```python
from build123d import *

# Parameters (mm, degrees)
F0_W     = 99
F0_H     = 38
F0_W_2   = 29.5
F0_H_2   = 16
F1_DEPTH = 3
F2_R     = 2.38125
F3_DEPTH = 3.001
F4_W     = 35.15
F4_H     = 22.55
F5_DEPTH = 1


with BuildPart() as f1:
    # F0 (on Top) → F1 (new body)
    with BuildSketch(Plane.XY):
        with Locations((49.5, 19)):
            Rectangle(F0_W, F0_H)
        with Locations((49.5, 19)):
            Rectangle(F0_W_2, F0_H_2, mode=Mode.SUBTRACT)
    extrude(amount=F1_DEPTH)

    # F2 (on face) → F3 (cut, through all)
    with BuildSketch(Plane.XY.offset(3)):
        with Locations((7.5, 19)):
            Circle(F2_R)
        with Locations((91.5, 19)):
            Circle(F2_R)
    extrude(amount=-F3_DEPTH, mode=Mode.SUBTRACT)

    # F4 (on face) → F5 (cut)
    with BuildSketch(Plane(origin=(0, 0, 0), x_dir=(1, 0, 0), z_dir=(0, 0, -1))):
        with Locations((49.5, -19)):
            Rectangle(F4_W, F4_H)
    extrude(amount=-F5_DEPTH, mode=Mode.SUBTRACT)


solid = f1.part
```
Part model, mm, in its own coordinate system. A direction names the side the tool comes from. Give positions to 0.01 mm unless a question says otherwise; leave off trailing zeros. Write each loop counter-clockwise with the first axis right and the second up, starting at its lowest first coordinate (ties: lowest second). Pieces come first, ordered by that corner, then holes. Notation, with made-up numbers: M -19.75,-22 L -12.75,-22 A20 cw -12.75,-15 Z; hole C 8,-31 d4. An arc over 180 degrees is marked long. Use CSV: the item, a comma, the result in double quotes.
Item 1: Slice it at B-B on x = 55.5. Write the cut outline in (y, z) (3 decimals), plus the area to 4 significant figures.
Taken from the geometry:
outline,"M 0,0 L 7.725,0 L 7.725,1 L 11,1 L 11,3 L 0,3 Z; M 27,1 L 30.275,1 L 30.275,0 L 38,0 L 38,3 L 27,3 Z"
area,"59.45 mm²"
Item 2: Slice it at C-C on y = 19. Write the cut outline in (x, z) (3 decimals), plus the area to 3 significant figures.
Taken from the geometry:
outline,"M 0,0 L 5.119,0 L 5.119,3 L 0,3 Z; M 9.881,0 L 31.925,0 L 31.925,1 L 34.75,1 L 34.75,3 L 9.881,3 Z; M 64.25,1 L 67.075,1 L 67.075,0 L 89.119,0 L 89.119,3 L 64.25,3 Z; M 93.881,0 L 99,0 L 99,3 L 93.881,3 Z"
area,"174 mm²"
Item 3: Slice it at D-D on x = 7.5. Write the cut outline in (y, z), plus the area to 3 significant figures.
Taken from the geometry:
outline,"M 0,0 L 16.62,0 L 16.62,3 L 0,3 Z; M 21.38,0 L 38,0 L 38,3 L 21.38,3 Z"
area,"99.7 mm²"
Item 4: Drill centre lines: probe 1 along Y at (x, z) = (7.5, 1.8); probe 2 along Y at (x, z) = (58, 0.75) (3 decimals); probe 3 along X at (y, z) = (15.5, 0.35) (3 decimals). Where is each one in solid material? Low to high.
Taken from the geometry:
probe 1,"y = 0 to 16.62, 21.38 to 38"
probe 2,"y = 0 to 7.725, 30.275 to 38"
probe 3,"x = 0 to 31.925, 67.075 to 99"
Item 5: Which spindle directions (+Z, -Z, +X, -X, +Y, -Y) get a long thin tool onto all of the face, cutting with end or side? Do faces 4 (the face through (0, 19, 1)), 5 (the face through (49, 9, 1)), 6 (the face through (49, 11, 2)). Say none if no direction does.
Taken from the geometry:
face 4,"+Z, -Z, -X, +Y, -Y"
face 5,"-Z"
face 6,"+Z, -Z"
Item 6: Pin check, flat tip, straight feed: P1, Ø0.8, axis at y = 24, z = 0.5, coming from the -X side. Stop position of the tip, or through.
Taken from the geometry:
P1,"stops at x = 0"
Item 7: Pull direction X, two halves, no side cores. Call faces 1 (the face through (48.8, 10.8, 3)), 2 (the face through (49, 27, 2)), 3 (the face through (99, 19, 1)): +X half, -X half, draft (parallel to the pull), parting line (faces both ways), or undercut.
Taken from the geometry:
face 1,"draft"
face 2,"undercut"
face 3,"+X half"
Item 8: Slice it at A-A on y = 13.5. Write the cut outline in (x, z) (3 decimals).
Taken from the geometry:
outline,"M 0,0 L 31.925,0 L 31.925,1 L 34.75,1 L 34.75,3 L 0,3 Z; M 64.25,1 L 67.075,1 L 67.075,0 L 99,0 L 99,3 L 64.25,3 Z"
